```python
from build123d import *

# Parameters (mm, degrees)
F0_W     = 22.5
F0_H     = 25
F1_DEPTH = 3
F2_R     = 2.05
F3_DEPTH = 25
F4_W     = 2
F4_H     = 2
F4_W_2   = 35.5
F5_DEPTH = 30
F7_DEPTH = 25
F8_R     = 2.1
F9_DEPTH = 25


with BuildPart() as f1:
    # F0 (on Top) → F1 (new body)
    with BuildSketch(Plane.XY):
        with Locations((11.25, 12.5)):
            Rectangle(F0_W, F0_H)
    extrude(amount=F1_DEPTH)

    # F2 (on face) → F3 (cut)
    with BuildSketch(Plane.XY.offset(3)):
        with Locations((9.25, 18)):
            Circle(F2_R)
        with Locations((13.25, 8)):
            Circle(F2_R)
    extrude(amount=-F3_DEPTH, mode=Mode.SUBTRACT)

    # F4 (on Top) → F5 (join)
    with BuildSketch(Plane.XY):
        with Locations((-14, 24)):
            Rectangle(F4_W, F4_H)
        with Locations((4.75, 24)):
            Rectangle(F4_W_2, F4_H)
        Polygon((-13, 23), (-15, 23), (-15, 11), (-14.244832817, 12.7950885872), (-13, 12.2714058573), align=None)
        Polygon((-14.244832817, 12.7950885872), (-15, 11), (-13, 11), (-13, 12.2714058573), align=None)
        Polygon((-13, 11), (-15, 11), (11.1478185281, 0), (11.9029857111, 1.7950885872), (-13, 12.2714058573), align=None)
    extrude(amount=-F5_DEPTH)

    # F6 (on Front) → F7 (cut)
    with BuildSketch(Plane.XZ):
        Polygon((22.5, -30), (22.5, -5.1932623562), (-15, -30), align=None)
    extrude(amount=-F7_DEPTH, mode=Mode.SUBTRACT)

    # F8 (on Right) → F9 (cut)
    with BuildSketch(Plane.YZ):
        with Locations((18, -5)):
            Circle(F8_R)
        with Locations((18, -25)):
            Circle(F8_R)
    extrude(amount=-F9_DEPTH, mode=Mode.SUBTRACT)


solid = f1.part
```
Check sheet for the modelled part. Datum: model origin and axes. Units: mm. A direction names the side the tool comes from. Coordinates: 2 decimals unless noted, no trailing zeros. Write each loop counter-clockwise with the first axis right and the second up, starting at its lowest first coordinate (ties: lowest second). Pieces come first, ordered by that corner, then holes. Notation, with made-up numbers: (77.5, 61.25) - (132.5, 61.25) arc R31 ccw to (132.5, 96.25) - close; hole circle Ø5 at (66.5, 34). An arc over 180 degrees is marked (long way). One line per question, with ' | ' between items.
Item 1: Access from +Z, -Z, +X, -X, +Y, -Y to the whole of each face (thin tool, end or side, straight path). Record for faces 4 (the face through (11.52, 0.88, -6.26)), 5 (the face through (11, 12, 0)), 6 (the face through (-14, 18, 0)).
Determined:
face 4: -Z, +X, -Y | face 5: -Z, +X | face 6: +Z, -X, +Y, -Y
Item 2: Gauge pin test, flat ends, axial feed: P1, Ø4.5, axis at x = -6, y = 13, coming from the +Z side; P2, Ø5, axis at x = 0, y = 5.5, coming from the -Z side; P3, Ø5, axis at x = -4.5, z = -9.5, coming from the -Y side; P4, Ø11, axis at x = 15, y = 12.5, coming from the -Z side. Record the tip position at first contact, or that the pin passes through.
Determined:
P1: passes through | P2: stops at z = -21.72 | P3: stops at y = 5.53 | P4: stops at z = 0
Item 3: Mould release check, pull along X, two halves, no side actions. Record for faces 1 (the face through (-13, 18, -14)), 2 (the face through (1, 23, -11)), 3 (the face through (11.2, 8.09, 1.52)): pulls with the +X half, pulls with the -X half, needs draft (parallel to the pull), parting line crosses it, or undercut.
Determined:
face 1: pulls with the +X half | face 2: needs draft | face 3: undercut
Item 4: Thickness scan on line 1 (Z direction, x = -14.2, y = 18); line 2 (Y direction, x = 17.5, z = -5); line 3 (Z direction, x = 8.5, y = 20). Record the ranges inside material, lowest first. Write a range as [from, to].
Determined:
line 1: z = [-29.47, -27.1], [-22.9, -7.1], [-2.9, 0] | line 2: y = [23, 25] | line 3: z = [0, 3]
Item 5: Sectioned sample at C-C on x = 9.25. Record the boundary of the cut face in (y, z), plus the area to 3 significant figures.
Determined:
outline: (0, 0) - (0.8, 0) - (0.8, -13.96) - (2.91, -13.96) - (2.91, 0) - (15.95, 0) - (15.95, 3) - (0, 3) - close; (20.05, 0) - (23, 0) - (23, -13.96) - (25, -13.96) - (25, 3) - (20.05, 3) - close | area: 120 mm2
Item 6: Sectioned sample at B-B on y = 12.75. Record the boundary of the cut face in (x, z), plus the area to 3 significant figures.
Determined:
outline: (-15, -30) - (-13, -28.68) - (-13, 0) - (-15, 0) - close; (0, 0) - (22.5, 0) - (22.5, 3) - (0, 3) - close | area: 126 mm2
Item 7: Sectioned sample at A-A on y = 18. Record the boundary of the cut face in (x, z).
Determined:
outline: (-15, -30) - (-13, -28.68) - (-13, -27.1) - (-15, -27.1) - close; (-15, -22.9) - (-13, -22.9) - (-13, -7.1) - (-15, -7.1) - close; (-15, -2.9) - (-13, -2.9) - (-13, 0) - (-15, 0) - close; (0, 0) - (7.2, 0) - (7.2, 3) - (0, 3) - close; (11.3, 0) - (22.5, 0) - (22.5, 3) - (11.3, 3) - close
Item 8: Sectioned sample at D-D on z = -6.5. Record the boundary of the cut face in (x, y), plus the area to 3 significant figures.
Determined:
outline: (-15, 11) - (11.15, 0) - (11.9, 1.8) - (-13, 12.27) - (-13, 16.53) - (-15, 16.53) - close; (-15, 19.47) - (-13, 19.47) - (-13, 23) - (20.52, 23) - (20.52, 25) - (-15, 25) - close | area: 142 mm2
